Autodesk Inventor part; units mm, degrees
ref_plane "YZ Plane" through (0, 0, 0) normal (1, 0, 0) x (0, 1, 0)
ref_plane "XZ Plane" through (0, 0, 0) normal (0, 1, 0) x (-1, 0, 0)
ref_plane "XY Plane" through (0, 0, 0) normal (0, 0, 1) x (1, 0, 0)
sketch "Sketch1" plane through (0, 0, 0) normal (1, 0, 0) x (0, 1, 0)
  line L0 (-7.62, 2.54) -> (0, 2.54)
  line L1 (0, 2.54) -> (0, 0)
  line L2 (0, 0) -> (-7.62, 0)
  line L3 (-7.62, 0) -> (-7.62, 2.54)
  line L4 (-7.62, 7.62) -> (-5.08, 7.62)
  line L5 (-5.08, 7.62) -> (-5.08, 2.54)
  line L6 (-5.08, 2.54) -> (-7.62, 2.54)
  line L7 (-7.62, 2.54) -> (-7.62, 7.62)
  line L8 (-1.27, 5.08) -> (0, 5.08)
  line L9 (0, 5.08) -> (0, 2.54)
  line L10 (0, 2.54) -> (-1.27, 2.54)
  line L11 (-1.27, 2.54) -> (-1.27, 5.08)
  dimension "d0" = 7.62
  dimension "d1" = 2.54
  dimension "d2" = 5.08
  dimension "d3" = 2.54
  dimension "d4" = 1.27
  dimension "d5" = 2.54
revolve "Revolution1" add sketch "Sketch1" angle 360 about axis through (0, 0, 2.54) along (0, 0, -1)
sketch "Sketch2" plane through (0, 0, 2.54) normal (0, 0, 1) x (1, 0, 0)
  circle A0 centre (-2.9748, -2.859) radius 0.3175
  line L0 (-0.6666, -1.081) -> (-1.7631, -2.859) construction
  line L1 (-1.7631, -2.859) -> (-2.9748, -2.859) construction
  circle A1 centre (0, 0) radius 1.27 construction
  circle A2 centre (-1.7631, -2.859) radius 0.3175
  point P0 (0, 0)
  dimension "d7" = 0.635
  dimension "d8" = 1.778
  dimension "d9" = 0.635
extrude "Extrusion1" cut sketch "Sketch2" along normal mid plane 25.4
sketch "Sketch3" plane through (0, 0, 2.54) normal (0, 0, 1) x (1, 0, 0)
  line L0 (0, 0) -> (1.8228, -2.926) construction
  line L1 (1.8228, -2.926) -> (3.0389, -2.926) construction
  line L2 (-1.5657, -3.1077) -> (1.8228, -2.926) construction
  circle A0 centre (-1.7631, -2.859) radius 0.3175
  circle A1 centre (1.8228, -2.926) radius 0.3175
  circle A2 centre (3.0389, -2.926) radius 0.3175
  circle A3 centre (1.962, 2.9682) radius 0.3175
  circle A4 centre (3.1781, 2.9682) radius 0.3175
  circle A5 centre (-1.2085, 2.832) radius 0.3175
  circle A6 centre (-2.506, 2.8679) radius 0.3175
  point P0 (0, 0)
  dimension "d12" = 0.635
  dimension "d13" = 0.635
  dimension "d14" = 0.635
  dimension "d15" = 0.635
  dimension "d16" = 0.635
  dimension "d17" = 0.635
extrude "Extrusion2" cut sketch "Sketch3" along normal mid plane 25.4 contours A1 | A2 | A3 | A4 | A5 | A6
sketch "Sketch4" plane through (0, 0, 2.54) normal (0, 0, 1) x (1, 0, 0)
  line L0 (-0.4549, -6.2616) -> (0.4549, -6.2616)
  line L1 (0.4549, -6.2616) -> (0.4549, 6.2616)
  line L2 (0.4549, 6.2616) -> (-0.4549, 6.2616)
  line L3 (-0.4549, 6.2616) -> (-0.4549, -6.2616)
  line L4 (-0.4549, -6.2616) -> (0.4549, 6.2616) construction
  line L5 (0.4549, -6.2616) -> (-0.4549, 6.2616) construction
  point P0 (0, 0)
  point P1 (0, 0)
extrude "Extrusion3" add sketch "Sketch4" along normal blind 5.08
sketch "Sketch5" plane through (0, 0, 2.54) normal (0, 0, 1) x (1, 0, 0)
  line L0 (-6.9573, 0.776) -> (6.9573, 0.776)
  line L1 (6.9573, 0.776) -> (6.9573, -0.776)
  line L2 (6.9573, -0.776) -> (-6.9573, -0.776)
  line L3 (-6.9573, -0.776) -> (-6.9573, 0.776)
  line L4 (-6.9573, 0.776) -> (6.9573, -0.776) construction
  line L5 (6.9573, 0.776) -> (-6.9573, -0.776) construction
  point P0 (0, 0)
  point P1 (0, 0)
extrude "Extrusion4" add sketch "Sketch5" along normal blind 3.302
properties part number "Mount"
Input: part model. Units: mm. Frame: model coordinates. A direction names the side the tool comes from. Give positions to 0.01 mm unless a question says otherwise; leave off trailing zeros. Loops run counter-clockwise (first coordinate to the right, second up) from the corner with the lowest first, then second, coordinate; pieces in that order, holes last. Notation, with made-up numbers: (46, -33.5) -> (59, -33.5) arc R30 cw to (59, -11.5) -> close; hole circle Ø2 at (4.25, -5). An arc over 180 degrees is marked (long way). Answer as a JSON object with one key per item and string values. Group by question number.
Item 1: Cut plane B-B, the plane x = -1.25. Return the cut outline in (y, z).
Item 2: Reachability of faces 1 (the flat face through (0, 0, 0)), 2 (the flat face through (2, 2, 2.54)) from +Z, -Z, +X, -X, +Y, -Y: full face, straight path, thin tool, end or side. Return the list, or none.
Item 3: Line query: probe 1 along X at (y, z) = (-3.5, 2.75); probe 2 along Y at (x, z) = (1.5, 5); probe 3 along Y at (x, z) = (4.25, 4). Output: solid intervals per line, ascending.
Item 4: Cut plane C-C, the plane y = 0. Return the cut outline in (x, z), and give its area (3 significant figures).
Item 5: Cut plane A-A, the plane z = 2.75. Return the cut outline in (x, y).
Item 6: Cut plane D-D, the plane z = 1.75. State how many separate pieces and enclosed holes the cut face has, and give its area (3 significant figures).
Item 7: Pin query (flat end, axial travel): P1, Ø1.7, axis at x = 3.5, z = 3.5, coming from the +Y side; P2, Ø2.5, axis at x = 3, z = 5, coming from the -Y side; P3, Ø0.5, axis at x = -2, y = 0, coming from the +Z side. Return the tip coordinate at first contact, or that it passes through.
Checks:
{
 "1": {"outline": "(-7.52, 0) -> (2.52, 0) -> (2.52, 2.54) -> (0.78, 2.54) -> (0.78, 5.84) -> (-0.78, 5.84) -> (-0.78, 2.54) -> (-4.92, 2.54) -> (-4.92, 7.62) -> (-7.52, 7.62) -> close; (3.15, 0) -> (7.52, 0) -> (7.52, 7.62) -> (4.92, 7.62) -> (4.92, 2.54) -> (3.15, 2.54) -> close"},
 "2": {"face 1": "-Z, +X, -X, +Y, -Y", "face 2": "+Z"},
 "3": {"probe 1": "x = -6.77 to -3.68, -0.45 to 0.45, 3.68 to 6.77", "probe 2": "y = -7.47 to -4.85, -0.78 to 0.78, 4.85 to 7.47", "probe 3": "y = -6.32 to -2.78, -0.78 to 0.78, 2.78 to 6.32"},
 "4": {"outline": "(-7.62, 0) -> (7.62, 0) -> (7.62, 7.62) -> (5.08, 7.62) -> (5.08, 5.84) -> (0.45, 5.84) -> (0.45, 7.62) -> (-0.45, 7.62) -> (-0.45, 5.84) -> (-5.08, 5.84) -> (-5.08, 7.62) -> (-7.62, 7.62) -> close", "area": "99.7 mm²"},
 "5": {"outline": "circle Ø15.24 at (0, 0); hole (-5.02, -0.78) arc R5.08 ccw to (-0.45, -5.06) -> (-0.45, -1.19) arc R1.27 cw to (-1.01, -0.78) -> close; hole (-5.02, 0.78) -> (-1.01, 0.78) arc R1.27 cw to (-0.45, 1.19) -> (-0.45, 5.06) arc R5.08 ccw to start; hole (0.45, -5.06) arc R5.08 ccw to (5.02, -0.78) -> (1.01, -0.78) arc R1.27 cw to (0.45, -1.19) -> close; hole (0.45, 1.19) arc R1.27 cw to (1.01, 0.78) -> (5.02, 0.78) arc R5.08 ccw to (0.45, 5.06) -> close"},
 "6": {"separate pieces": "1", "enclosed holes": "8", "area": "180 mm²"},
 "7": {"P1": "stops at y = 7.14", "P2": "stops at y = -7.42", "P3": "stops at z = 5.84"}
}
